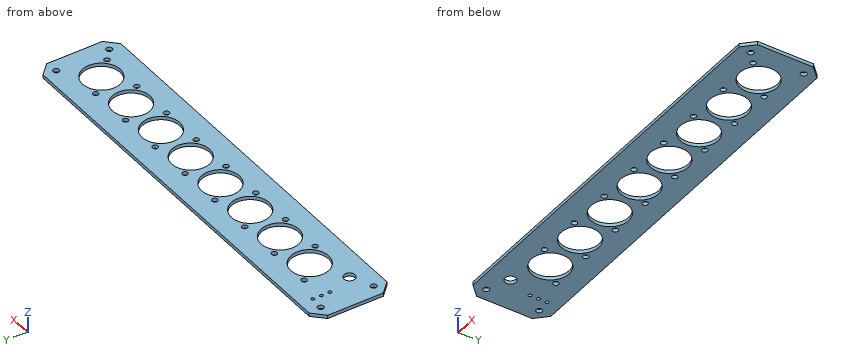
from build123d import *

# Parameters (mm, degrees)
F0_R     = 1.75
F0_R_2   = 3.25
F0_R_3   = 1.6
F0_R_4   = 1
F0_R_5   = 11
F1_DEPTH = 2


with BuildPart() as f1:
    # F0 (on Top) → F1 (new body)
    with BuildSketch(Plane.XY):
        Polygon((124.39022, 20.678444), (-108.10978, 20.678444), (-114.60978, 14.178444), (-114.60978, -18.321556), (-108.10978, -24.821556), (124.39022, -24.821556), (130.89022, -18.321556), (130.89022, 14.178444), align=None)
        with Locations((-107.35978, -17.571556)):
            Circle(F0_R, mode=Mode.SUBTRACT)
        with Locations((-94.60978, -11.971556)):
            Circle(F0_R_2, mode=Mode.SUBTRACT)
        with Locations((-64.70978, -11.971556)):
            Circle(F0_R_3, mode=Mode.SUBTRACT)
        with Locations((-38.70978, -11.971556)):
            Circle(F0_R_3, mode=Mode.SUBTRACT)
        with Locations((-12.70978, -11.971556)):
            Circle(F0_R_3, mode=Mode.SUBTRACT)
        with Locations((123.64022, -17.571556)):
            Circle(F0_R, mode=Mode.SUBTRACT)
        with Locations((13.29022, -11.971556)):
            Circle(F0_R_3, mode=Mode.SUBTRACT)
        with Locations((39.29022, -11.971556)):
            Circle(F0_R_3, mode=Mode.SUBTRACT)
        with Locations((65.29022, -11.971556)):
            Circle(F0_R_3, mode=Mode.SUBTRACT)
        with Locations((91.29022, -11.971556)):
            Circle(F0_R_3, mode=Mode.SUBTRACT)
        with Locations((117.29022, -11.971556)):
            Circle(F0_R_3, mode=Mode.SUBTRACT)
        with Locations((-99.60978, 2.828444)):
            Circle(F0_R_4, mode=Mode.SUBTRACT)
        with Locations((-74.60978, -2.071556)):
            Circle(F0_R_5, mode=Mode.SUBTRACT)
        with Locations((-99.60978, 7.828444)):
            Circle(F0_R_4, mode=Mode.SUBTRACT)
        with Locations((-84.50978, 7.828444)):
            Circle(F0_R_3, mode=Mode.SUBTRACT)
        with Locations((-58.50978, 7.828444)):
            Circle(F0_R_3, mode=Mode.SUBTRACT)
        with Locations((-48.60978, -2.071556)):
            Circle(F0_R_5, mode=Mode.SUBTRACT)
        with Locations((-22.60978, -2.071556)):
            Circle(F0_R_5, mode=Mode.SUBTRACT)
        with Locations((3.39022, -2.071556)):
            Circle(F0_R_5, mode=Mode.SUBTRACT)
        with Locations((-32.50978, 7.828444)):
            Circle(F0_R_3, mode=Mode.SUBTRACT)
        with Locations((-6.50978, 7.828444)):
            Circle(F0_R_3, mode=Mode.SUBTRACT)
        with Locations((-107.35978, 13.428444)):
            Circle(F0_R, mode=Mode.SUBTRACT)
        with Locations((-99.60978, 12.828444)):
            Circle(F0_R_4, mode=Mode.SUBTRACT)
        with Locations((29.39022, -2.071556)):
            Circle(F0_R_5, mode=Mode.SUBTRACT)
        with Locations((55.39022, -2.071556)):
            Circle(F0_R_5, mode=Mode.SUBTRACT)
        with Locations((19.49022, 7.828444)):
            Circle(F0_R_3, mode=Mode.SUBTRACT)
        with Locations((45.49022, 7.828444)):
            Circle(F0_R_3, mode=Mode.SUBTRACT)
        with Locations((81.39022, -2.071556)):
            Circle(F0_R_5, mode=Mode.SUBTRACT)
        with Locations((107.39022, -2.071556)):
            Circle(F0_R_5, mode=Mode.SUBTRACT)
        with Locations((71.49022, 7.828444)):
            Circle(F0_R_3, mode=Mode.SUBTRACT)
        with Locations((97.49022, 7.828444)):
            Circle(F0_R_3, mode=Mode.SUBTRACT)
        with Locations((123.64022, 13.428444)):
            Circle(F0_R, mode=Mode.SUBTRACT)
    extrude(amount=F1_DEPTH)


solid = f1.part
Input: part model. Units: mm. Frame: model coordinates. Give positions to 0.01 mm unless a question says otherwise; leave off trailing zeros. Loops run counter-clockwise (first coordinate to the right, second up) from the corner with the lowest first, then second, coordinate; pieces in that order, holes last. Notation, with made-up numbers: (-24.5, -34) - (-14.5, -34) arc R23 ccw to (-14.5, -24) - close; hole circle Ø2 at (-22.5, -11.5). An arc over 180 degrees is marked (long way). Use CSV: the item, a comma, the result in double quotes. Start each with the question number.
Item 1: Section B-B on x = 57. Return loops of the section in (y, z), then the cut area to 3 significant figures.
Item 2: Line query: line 1 (Y direction, x = 106.5, z = 1); line 2 (X direction, y = -19, z = 1.5); line 3 (X direction, y = 12, z = 1.05). Output: solid intervals per line, ascending.
Item 3: Contact query for flat-ended pins moving along their axis: P1, Ø5, axis at x = -41, y = 15, coming from the -Z side; P2, Ø1.6, axis at x = -99.61, y = 2.83, coming from the +Z side (1 decimal). Output: stop coordinate, or through.
Item 4: Section A-A on x = -16.5. Return loops of the section in (y, z), then the cut area to 3 significant figures.
Item 5: Section C-C on z = 1.2. State how many separate pieces and enclosed holes the cut face has, then the cut area to 3 significant figures.
Ans:
1,outline,"(-24.82, 0) - (-12.95, 0) - (-12.95, 2) - (-24.82, 2) - close; (8.81, 0) - (20.68, 0) - (20.68, 2) - (8.81, 2) - close"
1,area,"47.5 mm2"
2,line 1,"y = -24.82 to -13.04, 8.89 to 20.68"
2,line 2,"x = -113.93 to -108.37, -106.35 to 122.63, 124.65 to 130.21"
2,line 3,"x = -114.61 to -108.37, -106.35 to -100.17, -99.05 to 122.63, 124.65 to 130.89"
3,P1,"stops at z = 0"
3,P2,"passes through"
4,outline,"(-24.82, 0) - (-11.22, 0) - (-11.22, 2) - (-24.82, 2) - close; (7.08, 0) - (20.68, 0) - (20.68, 2) - (7.08, 2) - close"
4,area,"54.4 mm2"
5,separate pieces,"1"
5,enclosed holes,"32"
5,area,"7,830 mm2"
